from build123d import *

# Parameters (mm, degrees)
MODEL_R             = 9.8
MODEL_R_2           = 6
MODEL_W             = 15
MODEL_H             = 30
BOSS_EXTRUDE1_DEPTH = 3


with BuildPart() as part:
    # Model → Boss-Extrude1 (new body)
    with BuildSketch(Plane.XY):
        Polygon((-160.191927583, -27), (-160.191927583, -57), (-157.191927583, -57), (-157.191927583, -87), (-277.191927583, -87), (-277.191927583, -57), (-280.191927583, -57), (-280.191927583, -27), (-277.191927583, -27), (-277.191927583, 3), (-269.191927583, 3), (-269.191927583, 0), (-259.191927583, 0), (-259.191927583, 3), (-178.191927583, 3), (-178.191927583, 0), (-168.191927583, 0), (-168.191927583, 3), (-157.191927583, 3), (-157.191927583, -27), align=None)
        with Locations((-238.191927583, -68)):
            Circle(MODEL_R, mode=Mode.SUBTRACT)
        with Locations((-199.191927583, -68)):
            Circle(MODEL_R_2, mode=Mode.SUBTRACT)
        with Locations((-182.691927583, -42)):
            Rectangle(MODEL_W, MODEL_H, mode=Mode.SUBTRACT)
        with BuildLine():
            Line((-235.363500459, -40), (-230.191927583, -40))
            Line((-230.191927583, -40), (-230.191927583, -38))
            Line((-230.191927583, -38), (-246.191927583, -38))
            Line((-246.191927583, -38), (-246.191927583, -40))
            Line((-246.191927583, -40), (-241.020354708, -40))
            ThreePointArc((-241.020354708, -40), (-238.191927583, -44), (-235.363500459, -40))
        make_face(mode=Mode.SUBTRACT)
    extrude(amount=BOSS_EXTRUDE1_DEPTH)


solid = part.part
Part model, mm, in its own coordinate system. A direction names the side the tool comes from. Give positions to 0.01 mm unless a question says otherwise; leave off trailing zeros. Order: outer loops, then holes, each group sorted by start corner. A loop starts at its lowest first (then second) coordinate and runs counter-clockwise, first axis right, second up. Notation, with made-up numbers: (15.5, -38) - (21.5, -38) arc R15 ccw to (21.5, -21) - close; hole circle Ø3 at (-14, 75.25). An arc over 180 degrees is marked (long way). Use a Markdown table: item, result.
1) Two-plate mould, pull along Y, no slides. Class faces 1 (the flat face through (-219, 3, 1)), 2 (the flat face through (-160.192, -42, 1)), 3 (the flat face through (-259.192, 1, 1)): +Y half, -Y half, draft (parallel to the pull), parting line (faces both ways), or undercut.
Checked values:
| item | result |
|---|---|
| face 1 | +Y half |
| face 2 | undercut |
| face 3 | draft |
2) Saw through at C-C on y = -54. List the corners of the cut face in (x, z).
Checked values:
| item | result |
|---|---|
| outline | (-280.19, 0) - (-190.19, 0) - (-190.19, 3) - (-280.19, 3) - close; (-175.19, 0) - (-160.19, 0) - (-160.19, 3) - (-175.19, 3) - close |
3) Saw through at A-A on y = -68. List the corners of the cut face in (x, z), plus the area to 3 significant figures.
Checked values:
| item | result |
|---|---|
| outline | (-277.19, 0) - (-247.99, 0) - (-247.99, 3) - (-277.19, 3) - close; (-228.39, 0) - (-205.19, 0) - (-205.19, 3) - (-228.39, 3) - close; (-193.19, 0) - (-157.19, 0) - (-157.19, 3) - (-193.19, 3) - close |
| area | 265 mm² |
4) Flat gauge pins, fed straight in: P1, Ø1.5, axis at x = -279, z = 1.5, coming from the +Y side; P2, Ø0.9, axis at y = -8, z = 1, coming from the -X side; P3, Ø12, axis at x = -189, y = -52.5, coming from the -Z side; P4, Ø1.5, axis at x = -265.5, z = 1.5, coming from the +Y side. Where does each tip first touch, or does it go through?
Checked values:
| item | result |
|---|---|
| P1 | y = -27 |
| P2 | x = -277.19 |
| P3 | z = 0 |
| P4 | y = 0 |
5) 3-axis set-ups, long thin cutter, end or side, ignore diameter. For faces 4 (the flat face through (-279, -27, 1)), 5 (the flat face through (-159, -27, 1)), 6 (the flat face through (-183, -27, 1)): which of +Z, -Z, +X, -X, +Y, -Y reach the whole face in a straight line?
Checked values:
| item | result |
|---|---|
| face 4 | +Z, -Z, -X, +Y |
| face 5 | +Z, -Z, +X |
| face 6 | +Z, -Z |
6) Probe L1, parallel to X at y = -41, z = 0.9; L2, parallel to Y at x = -244.5, z = 2.1; L3, parallel to Y at x = -235, z = 2.7. List the from-to ranges inside material, lowest first. Write a range as from..to.
Checked values:
| item | result |
|---|---|
| L1 | -280.19..-241.19, -235.19..-190.19, -175.19..-160.19 |
| L2 | -87..-75.5, -60.5..-40, -38..3 |
| L3 | -87..-77.27, -58.73..-40, -38..3 |
7) Saw through at D-D on z = 1.8. Count the separate pieces of the cut face and the enclosed holes in it, plus the area to 3 significant figures.
Checked values:
| item | result |
|---|---|
| separate pieces | 1 |
| enclosed holes | 4 |
| area | 9,820 mm² |
8) Saw through at B-B on x = -181.5. List the corners of the cut face in (y, z).
Checked values:
| item | result |
|---|---|
| outline | (-87, 0) - (-57, 0) - (-57, 3) - (-87, 3) - close; (-27, 0) - (3, 0) - (3, 3) - (-27, 3) - close |
